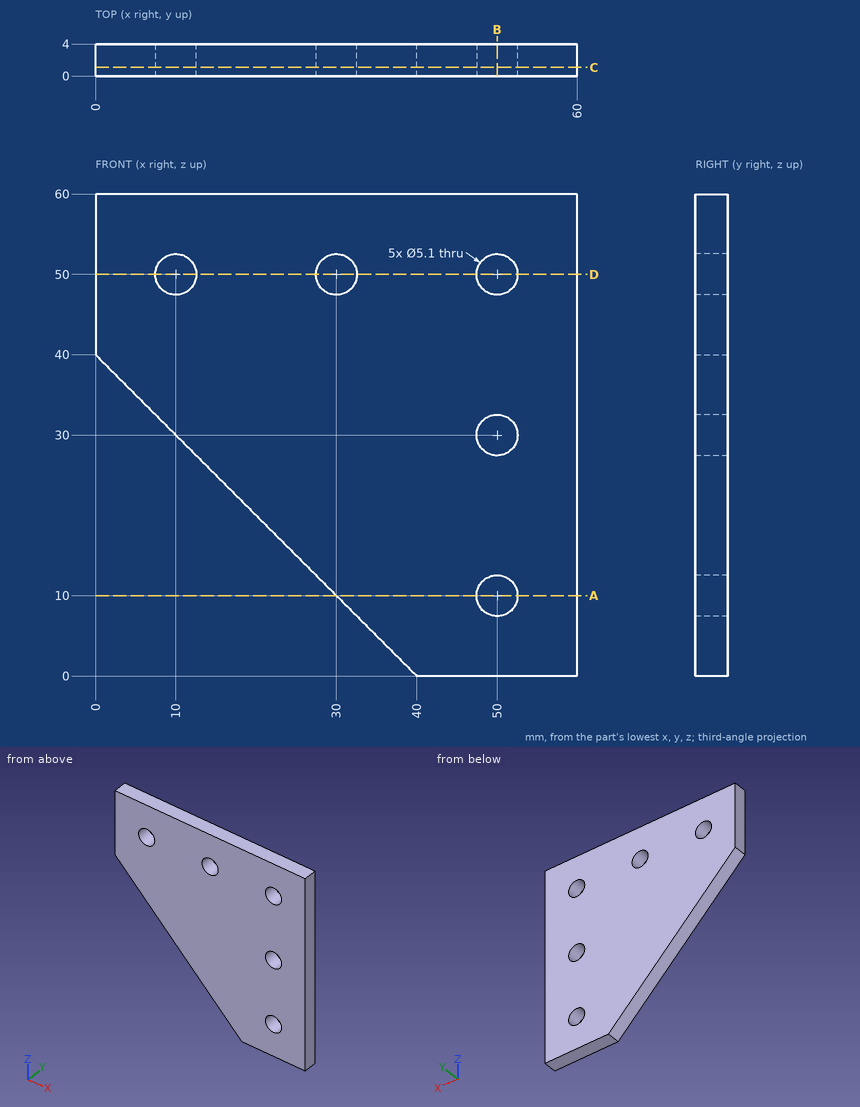
Source: three-view drawing plus pictorial views. Frame: mm from the lowest corner of the part. Give positions to 0.01 mm unless a question says otherwise; leave off trailing zeros. Write each loop counter-clockwise with the first axis right and the second up, starting at its lowest first coordinate (ties: lowest second). Pieces come first, ordered by that corner, then holes. Notation, with made-up numbers: (17, -34) - (74, -34) arc R23 ccw to (74, -16) - close; hole circle Ø4 at (69.5, 76.5). An arc over 180 degrees is marked (long way). Write item = value, one per line. Start each with the question number.
1. Section query A-A, the plane z = 10. Output: boundary loops of the cut face in (x, y), then the cut area to 3 significant figures.
2. First-contact query: pin 1 Ø1.5 at (x, y) = (35.5, 3) entering from -Z; pin 2 Ø8 at (x, z) = (50, 30) entering from +Y; pin 3 Ø2 at (y, z) = (1.5, 27.5) entering from -X; pin 4 Ø1 at (x, y) = (23.5, 0.5) entering from -Z. Flat tips, straight axial feed; report the tip coordinate or a pass-through.
3. Ray query, L1, parallel to Z at x = 50, y = 1.5; L2, parallel to Z at x = 10, y = 1.6; L3, parallel to Z at x = 51.5, y = 0.55. Return the intervals inside material, ascending.
4. Section query B-B, the plane x = 50. Output: boundary loops of the cut face in (y, z), then the cut area to 3 significant figures.
5. Section query C-C, the plane y = 1.1. Output: boundary loops of the cut face in (x, z), then the cut area to 3 significant figures.
6. Section query D-D, the plane z = 50. Output: boundary loops of the cut face in (x, y), then the cut area to 3 significant figures.
Check sheet entries:
q1.outline = (30, 0) - (47.45, 0) - (47.45, 4) - (30, 4) - close; (52.55, 0) - (60, 0) - (60, 4) - (52.55, 4) - close
q1.area = 99.6 mm2
q2.pin_1 = 3.75
q2.pin_2 = 4
q2.pin_3 = 11.5
q2.pin_4 = 16
q3.L1 = 0 to 7.45, 12.55 to 27.45, 32.55 to 47.45, 52.55 to 60
q3.L2 = 30 to 47.45, 52.55 to 60
q3.L3 = 0 to 7.94, 12.06 to 27.94, 32.06 to 47.94, 52.06 to 60
q4.outline = (0, 0) - (4, 0) - (4, 7.45) - (0, 7.45) - close; (0, 12.55) - (4, 12.55) - (4, 27.45) - (0, 27.45) - close; (0, 32.55) - (4, 32.55) - (4, 47.45) - (0, 47.45) - close; (0, 52.55) - (4, 52.55) - (4, 60) - (0, 60) - close
q4.area = 179 mm2
q5.outline = (0, 40) - (40, 0) - (60, 0) - (60, 60) - (0, 60) - close; hole circle Ø5.1 at (10, 50); hole circle Ø5.1 at (30, 50); hole circle Ø5.1 at (50, 10); hole circle Ø5.1 at (50, 30); hole circle Ø5.1 at (50, 50)
q5.area = 2,700 mm2
q6.outline = (0, 0) - (7.45, 0) - (7.45, 4) - (0, 4) - close; (12.55, 0) - (27.45, 0) - (27.45, 4) - (12.55, 4) - close; (32.55, 0) - (47.45, 0) - (47.45, 4) - (32.55, 4) - close; (52.55, 0) - (60, 0) - (60, 4) - (52.55, 4) - close
q6.area = 179 mm2
